Geometry check sheet. Reference: the model listing, model coordinates, mm. A direction names the side the tool comes from. Coordinates: 2 decimals unless noted, no trailing zeros. Write each loop counter-clockwise with the first axis right and the second up, starting at its lowest first coordinate (ties: lowest second). Pieces come first, ordered by that corner, then holes. Notation, with made-up numbers: M 21,-23 L 53,-23 A30 ccw 53,13 Z; hole C 48.25,53.5 d1. An arc over 180 degrees is marked long. Answer as a JSON object with one key per item and string values. Group by question number.
```python
from build123d import *

# Parameters (mm, degrees)
F1_DEPTH = 40
F2_R     = 2.15
F3_DEPTH = 1
F4_R     = 5


with BuildPart() as f1:
    # F0 (on Front) → F1 (new body, symmetric)
    with BuildSketch(Plane.XZ):
        with BuildLine():
            Line((0, 1), (0, 0))
            Line((0, 0), (17.7, 0))
            ThreePointArc((17.7, 0), (19.326346, 0.673654), (20, 2.3))
            Line((20, 2.3), (20, 13.7))
            ThreePointArc((20, 13.7), (20.380761, 14.619239), (21.3, 15))
            Line((21.3, 15), (28, 15))
            Line((28, 15), (28, 16))
            Line((28, 16), (21.3, 16))
            ThreePointArc((21.3, 16), (19.673654, 15.326346), (19, 13.7))
            Line((19, 13.7), (19, 2.3))
            ThreePointArc((19, 2.3), (18.619239, 1.380761), (17.7, 1))
            Line((17.7, 1), (0, 1))
        make_face()
    extrude(amount=F1_DEPTH, both=True)

    # F2 (on face) → F3 (cut, through all)
    with BuildSketch(Plane.XY.offset(1)):
        with Locations((8, 25)):
            Circle(F2_R)
        with Locations((8, 0)):
            Circle(F2_R)
        with Locations((8, -25)):
            Circle(F2_R)
    extrude(amount=-F3_DEPTH, mode=Mode.SUBTRACT)

    # F4
    f4_edges = [f1.edges().sort_by_distance(p)[0] for p in [
        (0, 40, 0.5),
        (0, -40, 0.5),
        (28, -40, 15.5),
        (28, 40, 15.5),
    ]]
    fillet(f4_edges, radius=F4_R)


solid = f1.part
```
1) Section check B-B (z = 5.75). Record the cut outline in (x, y), then the cut area to 3 significant figures.
2) Material ranges on probe 1 along Y at (x, z) = (8, 0.35); probe 2 along X at (y, z) = (-2.5, 6.25); probe 3 along Z at (x, y) = (12, 29), recorded low to high. Write a range as [from, to].
3) Draft check along X on faces 4 (the cylindrical face through (19.31, -0.56, 0.66)), 5 (the cylindrical face through (1.43, -38.5, 0.49)), 6 (the cylindrical face through (10.05, 0.65, 0.51)). Enter one of: +X half, -X half, draft (parallel to the pull), parting line (faces both ways), or undercut.
4) Section check A-A (y = 25). Record the cut outline in (x, z), then the cut area to 3 significant figures.
5) Go/stop test with flat-tipped pins: pin 1 Ø3 at (y, z) = (-1, 8.5) entering from -X; pin 2 Ø3 at (x, z) = (16.5, 12.5) entering from -Y; pin 3 Ø3.5 at (y, z) = (18.5, 7.5) entering from +X; pin 4 Ø7.5 at (x, y) = (24.5, -1) entering from -Z. Record where each tip stops, or that it passes through.
6) Set-up check for faces 1 (the flat face through (25, -1, 15)), 2 (the flat face through (11, -1, 1)), 3 (the flat face through (19.3, 40, 5.7)): record each of +Z, -Z, +X, -X, +Y, -Y from which the full face is reachable in a straight line by a thin tool's end or side.
7) Section check C-C (x = 15.25). Record the cut outline in (y, z).
Entries:
{
 "1": {"outline": "M 19,-40 L 20,-40 L 20,40 L 19,40 Z", "area": "80.0 mm^2"},
 "2": {"probe 1": "[-40, -27.15], [-22.85, -2.15], [2.15, 22.85], [27.15, 40]", "probe 2": "[19, 20]", "probe 3": "[0, 1]"},
 "3": {"face 4": "+X half", "face 5": "-X half", "face 6": "undercut"},
 "4": {"outline": "M 0,0 L 5.85,0 L 5.85,1 L 0,1 Z; M 10.15,0 L 17.7,0 A2.3 ccw 20,2.3 L 20,13.7 A1.3 cw 21.3,15 L 28,15 L 28,16 L 21.3,16 A2.3 ccw 19,13.7 L 19,2.3 A1.3 cw 17.7,1 L 10.15,1 Z", "area": "37.2 mm^2"},
 "5": {"pin 1": "x = 19", "pin 2": "through", "pin 3": "x = 20", "pin 4": "z = 14.88"},
 "6": {"face 1": "-Z, +X, +Y, -Y", "face 2": "+Z, -X, +Y, -Y", "face 3": "+Z, -Z, +X, -X, +Y"},
 "7": {"outline": "M -40,0 L 40,0 L 40,1 L -40,1 Z"}
}
